from build123d import *

# Parameters (mm, degrees)
RESSALTO_EXTRUS_O2_DEPTH = 10
ESBO_O4_W                = 2.6
ESBO_O4_H                = 3.2
CORTE_EXTRUS_O1_DEPTH    = 5
CHANFRO2_SIZE            = 0.5
CHANFRO3_SIZE            = 0.5
ESBO_O10_R               = 0.35
RESSALTO_EXTRUS_O5_DEPTH = 3.6
CHANFRO4_SIZE            = 0.3


with BuildPart() as part:
    # Esboço2 → Ressalto-extrusão2 (new body)
    with BuildSketch(Plane.XY):
        with BuildLine():
            Line((0, 0), (10.4, 0))
            Line((10.4, 0), (10.4, 7))
            ThreePointArc((10.4, 7), (10.107106781, 7.707106781), (9.4, 8))
            Line((9.4, 8), (8.35, 14.4))
            Line((8.35, 14.4), (5.2, 14.4))
            Line((5.2, 14.4), (2.05, 14.4))
            Line((2.05, 14.4), (0, 5))
            Line((0, 5), (0, 0))
        make_face()
    extrude(amount=-RESSALTO_EXTRUS_O2_DEPTH)

    # Esboço4 → Corte-extrusão1 (cut)
    with BuildSketch(Plane(origin=(10.4, 0, 0), x_dir=(0, 0, -1), z_dir=(1, 0, 0))):
        with Locations((2.6, 3.6)):
            Rectangle(ESBO_O4_W, ESBO_O4_H)
        with Locations((7.4, 3.6)):
            Rectangle(ESBO_O4_W, ESBO_O4_H)
    extrude(amount=-CORTE_EXTRUS_O1_DEPTH, mode=Mode.SUBTRACT)

    # Chanfro2
    chanfro2_edges = [part.edges().sort_by_distance(p)[0] for p in [
        (10.4, 3.6, -1.3),
        (10.4, 2, -2.6),
        (10.4, 3.6, -3.9),
        (10.4, 5.2, -2.6),
    ]]
    chamfer(chanfro2_edges, length=CHANFRO2_SIZE)

    # Chanfro3
    chanfro3_edges = [part.edges().sort_by_distance(p)[0] for p in [
        (10.4, 3.6, -8.7),
        (10.4, 5.2, -7.4),
        (10.4, 3.6, -6.1),
        (10.4, 2, -7.4),
    ]]
    chamfer(chanfro3_edges, length=CHANFRO3_SIZE)

    # Esboço10 → Ressalto-extrusão5 (add)
    with BuildSketch(Plane.XZ):
        with Locations(Location((4.3, -2.2, 0), (0, 0, 270))):
            Circle(ESBO_O10_R)
        with Locations(Location((4.3, -7.8, 0), (0, 0, 270))):
            Circle(ESBO_O10_R)
    extrude(amount=RESSALTO_EXTRUS_O5_DEPTH)

    # Chanfro4
    chanfro4_edges = [part.edges().sort_by_distance(p)[0] for p in [
        (4.3, -3.6, -1.85),
        (4.3, -3.6, -7.45),
    ]]
    chamfer(chanfro4_edges, length=CHANFRO4_SIZE)


solid = part.part
Geometry check sheet. Reference: the model listing, model coordinates, mm. A direction names the side the tool comes from. Give positions to 0.01 mm unless a question says otherwise; leave off trailing zeros. Write each loop counter-clockwise with the first axis right and the second up, starting at its lowest first coordinate (ties: lowest second). Pieces come first, ordered by that corner, then holes. Notation, with made-up numbers: (53, 79) - (60, 79) arc R34 ccw to (60, 116) - close; hole circle Ø10 at (81, 32.25). An arc over 180 degrees is marked (long way). Put each result on its own line as item: value.
1. Sectioned sample at B-B, the plane x = 7.25. Enter the section's corners in (y, z).
Ans:
outline: (0, -10) - (14.4, -10) - (14.4, 0) - (0, 0) - close; hole (2, -8.7) - (5.2, -8.7) - (5.2, -6.1) - (2, -6.1) - close; hole (2, -3.9) - (5.2, -3.9) - (5.2, -1.3) - (2, -1.3) - close
2. Thickness scan on line 1 (Z direction, x = 9, y = 3); line 2 (Y direction, x = 8, z = -1.5); line 3 (X direction, y = 2.5, z = -3.5). Record the ranges inside material, lowest first.
Ans:
line 1: z = -10 to -8.7, -6.1 to -3.9, -1.3 to 0
line 2: y = 0 to 2, 5.2 to 14.4
line 3: x = 0 to 5.4
3. Draft check along Z on faces 3 (the flat face through (5, 7, 0)), 4 (the flat face through (5.4, 4, -7)), 5 (the flat face through (8.88, 11.16, -4.93)), 6 (the flat face through (8, 4, -3.9)). Enter one of: +Z half, -Z half, draft (parallel to the pull), parting line (faces both ways), or undercut.
Ans:
face 3: +Z half
face 4: undercut
face 5: draft
face 6: undercut
4. Sectioned sample at A-A, the plane y = 2.75. Enter the section's corners in (x, z), plus the area to 3 significant figures.
Ans:
outline: (0, -10) - (10.4, -10) - (10.4, -9.2) - (9.9, -8.7) - (5.4, -8.7) - (5.4, -6.1) - (9.9, -6.1) - (10.4, -5.6) - (10.4, -4.4) - (9.9, -3.9) - (5.4, -3.9) - (5.4, -1.3) - (9.9, -1.3) - (10.4, -0.8) - (10.4, 0) - (0, 0) - close
area: 77.5 mm²
5. Sectioned sample at D-D, the plane y = 6. Enter the section's corners in (x, z).
Ans:
outline: (0.22, -10) - (10.4, -10) - (10.4, 0) - (0.22, 0) - close
6. Sectioned sample at C-C, the plane x = 1.5. Enter the section's corners in (y, z).
Ans:
outline: (0, -10) - (11.88, -10) - (11.88, 0) - (0, 0) - close
7. Go/stop test with flat-tipped pins: pin 1 (0.8 mm diameter, centred on y = 4, z = -8, fed in from +X); pin 2 (3 mm diameter, centred on x = 7.5, z = -7.5, fed in from -Y); pin 3 (6 mm diameter, centred on y = 12, z = -6.5, fed in from -X). Record where each tip stops, or that it passes through.
Ans:
pin 1: stops at x = 5.4
pin 2: stops at y = 0
pin 3: stops at x = 0.87
8. Set-up check for faces 1 (the flat face through (10.4, 3, -5)), 2 (the flat face through (5.4, 4, -3)): record each of +Z, -Z, +X, -X, +Y, -Y from which the full face is reachable in a straight line by a thin tool's end or side.
Ans:
face 1: +Z, -Z, +X, +Y, -Y
face 2: +X
